Geometry check sheet. Reference: the model listing, model coordinates, mm. Face numbers are marked on the shaded views. A direction names the side the tool comes from. Coordinates: 2 decimals unless noted, no trailing zeros. Write each loop counter-clockwise with the first axis right and the second up, starting at its lowest first coordinate (ties: lowest second). Pieces come first, ordered by that corner, then holes. Notation, with made-up numbers: (65.25, 32) -> (97.25, 32) arc R14 ccw to (97.25, 48) -> close; hole circle Ø10 at (27, 46). An arc over 180 degrees is marked (long way). Answer as CSV lines item,"result".
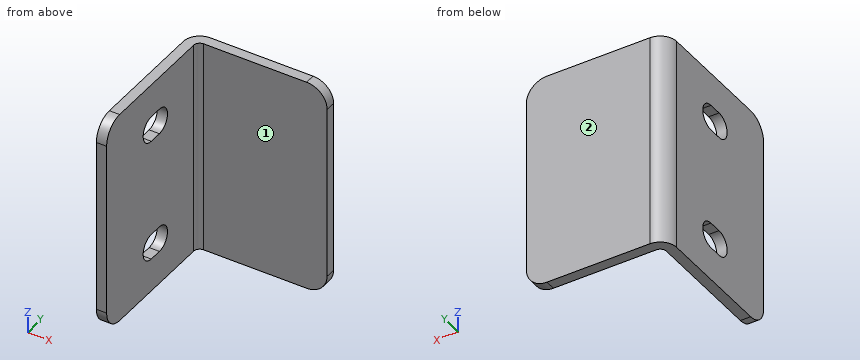
```python
from build123d import *

# Parameters (mm, degrees)
SKETCH1_W          = 24
SKETCH1_H          = 42
BASE_FLANGE1_DEPTH = 2
EDGE_FLANGE1_DEPTH = 42
FILLET1_R          = 4
CUT_EXTRUDE1_DEPTH = 2


# Sheet-metal steps are written as plain solids
with BuildPart() as part:
    # Sketch1 → Base-Flange1 (new body)
    with BuildSketch(Plane(origin=(0, 0, 0), x_dir=(1, 0, 0), z_dir=(0, 1, 0))):
        Rectangle(SKETCH1_W, SKETCH1_H)
    extrude(amount=BASE_FLANGE1_DEPTH)

    # Edge-Flange1 section (across the edge) → Edge-Flange1 (add)
    with BuildSketch(Plane(origin=(-13.2, 0, 21), x_dir=(1, 0, 0), z_dir=(0, 0, -1))):
        with BuildLine():
            Line((-2, 1.2), (-2, 28))
            Line((-2, 28), (0, 28))
            Line((0, 28), (0, 1.2))
            ThreePointArc((0, 1.2), (0.351471863, 0.351471863), (1.2, 0))
            Line((1.2, 0), (1.2, -2))
            ThreePointArc((1.2, -2), (-1.0627417, -1.0627417), (-2, 1.2))
        make_face()
    extrude(amount=EDGE_FLANGE1_DEPTH)

    # Fillet1
    fillet1_edges = [part.edges().sort_by_distance(p)[0] for p in [
        (-14.2, -28, 21),
        (-14.2, -28, -21),
        (12, 1, 21),
        (12, 1, -21),
    ]]
    fillet(fillet1_edges, radius=FILLET1_R)

    # Sketch11 → Cut-Extrude1 (cut)
    with BuildSketch(Plane(origin=(-13.2, 0, 0), x_dir=(0, 0, -1), z_dir=(1, 0, 0))):
        with BuildLine():
            Line((9.5, -14.25), (9.5, -11.75))
            ThreePointArc((9.5, -11.75), (12, -9.25), (14.5, -11.75))
            Line((14.5, -11.75), (14.5, -14.25))
            ThreePointArc((14.5, -14.25), (12, -16.75), (9.5, -14.25))
        make_face()
        with BuildLine():
            Line((-9.5, -14.25), (-9.5, -11.75))
            ThreePointArc((-9.5, -11.75), (-12, -9.25), (-14.5, -11.75))
            Line((-14.5, -11.75), (-14.5, -14.25))
            ThreePointArc((-14.5, -14.25), (-12, -16.75), (-9.5, -14.25))
        make_face()
    extrude(amount=-CUT_EXTRUDE1_DEPTH, mode=Mode.SUBTRACT)


solid = part.part
```
Item 1: Set-up check for the marked faces 1 and 2: record each of +Z, -Z, +X, -X, +Y, -Y from which the full face is reachable in a straight line by a thin tool's end or side.
Responses:
face 1,"+Z, -Z, +X, -Y"
face 2,"+Z, -Z, +X, -X, +Y"
Item 2: Cross-section at A-A, the plane z = 12. Record the cut outline in (x, y), plus the area to 3 significant figures.
Responses:
outline,"(-15.2, -28) -> (-13.2, -28) -> (-13.2, -16.75) -> (-15.2, -16.75) -> close; (-15.2, -9.25) -> (-13.2, -9.25) -> (-13.2, -1.2) arc R1.2 cw to (-12, 0) -> (12, 0) -> (12, 2) -> (-12, 2) arc R3.2 ccw to (-15.2, -1.2) -> close"
area,"93.5 mm2"
Item 3: Thickness scan on probe 1 along X at (y, z) = (-22, 5); probe 2 along Y at (x, z) = (-4.5, -8); probe 3 along Z at (x, y) = (-14, -24.75). Record the ranges inside material, lowest first.
Responses:
probe 1,"x = -15.2 to -13.2"
probe 2,"y = 0 to 2"
probe 3,"z = -20.93 to 20.93"
Item 4: Cross-section at D-D, the plane x = -11.5. Record the cut outline in (y, z).
Responses:
outline,"(0, -21) -> (2, -21) -> (2, 21) -> (0, 21) -> close"
Item 5: Depth check by flat-ended pin: pin 1 Ø3 at (y, z) = (-3, -9) entering from +X; pin 2 Ø5 at (x, z) = (5, -2.5) entering from -Y. Enter the tip coordinate at first touch or a pass-through.
Responses:
pin 1,"stops at x = -13.2"
pin 2,"stops at y = 0"
Item 6: Cross-section at B-B, the plane z = 5.5. Record the cut outline in (x, y), plus the area to 3 significant figures.
Responses:
outline,"(-15.2, -28) -> (-13.2, -28) -> (-13.2, -1.2) arc R1.2 cw to (-12, 0) -> (12, 0) -> (12, 2) -> (-12, 2) arc R3.2 ccw to (-15.2, -1.2) -> close"
area,"109 mm2"
Item 7: Cross-section at C-C, the plane y = -5. Record the cut outline in (x, z), plus the area to 3 significant figures.
Responses:
outline,"(-15.2, -21) -> (-13.2, -21) -> (-13.2, 21) -> (-15.2, 21) -> close"
area,"84.0 mm2"
